```python
from build123d import *

# Parameters (mm, degrees)
F0_R     = 7.5
F0_R_2   = 6.5
F1_DEPTH = 70
F2_R     = 8
F3_DEPTH = 100
F4_R     = 2


with BuildPart() as f1:
    # F0 (on Top) → F1 (new body)
    with BuildSketch(Plane.XY):
        Circle(F0_R)
        Circle(F0_R_2, mode=Mode.SUBTRACT)
    extrude(amount=F1_DEPTH)

    # F2 (on face) → F3 (join)
    with BuildSketch(Plane(origin=(0, 0, 0), x_dir=(1, 0, 0), z_dir=(0, 0, -1))):
        Circle(F2_R)
    extrude(amount=F3_DEPTH)

    # F4
    f4_edges = [f1.edges().sort_by_distance(p)[0] for p in [
        (-8, 0, -100),
    ]]
    fillet(f4_edges, radius=F4_R)


solid = f1.part
```
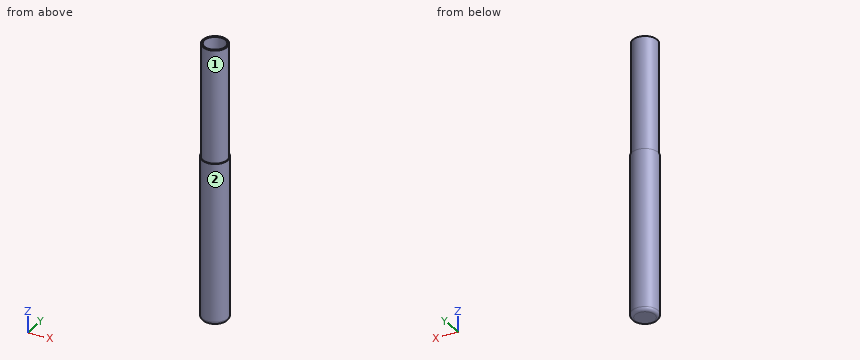
Input: part model. Units: mm. Frame: model coordinates. Face numbers are marked on the shaded views. A direction names the side the tool comes from. Coordinates: 2 decimals unless noted, no trailing zeros. Loops run counter-clockwise (first coordinate to the right, second up) from the corner with the lowest first, then second, coordinate; pieces in that order, holes last.
Q1. Contact query for flat-ended pins moving along their axis: pin 1 (1 mm diameter, centred on y = 4, z = -83, fed in from -X); pin 2 (1.5 mm diameter, centred on x = -3, z = 34, fed in from -Y); pin 3 (2 mm diameter, centred on x = 6, z = -53, fed in from +Y) (3 decimals). Output: stop coordinate, or through.
Results are:
pin 1: stops at x = -7.19
pin 2: stops at y = -7.15
pin 3: stops at y = 6.245
Q2. Line query: line 1 along Y through (x, z) = (0, 14); line 2 along Z through (x, y) = (3.5, -2); line 3 along X through (y, z) = (-2.25, 20). Output: solid intervals per line, ascending.
Results are:
line 1: y = -7.5 to -6.5, 6.5 to 7.5
line 2: z = -100 to 0
line 3: x = -7.15 to -6.1, 6.1 to 7.15
Q3. Section C-C, the plane z = 30. Return the cut outline in (x, y), and give its area (3 significant figures).
Results are:
outline: circle Ø15 at (0, 0); hole circle Ø13 at (0, 0)
area: 44.0 mm2
Q4. Section A-A, the plane x = 0. Return the cut outline in (y, z).
Results are:
outline: (-8, -98) arc R2 ccw to (-6, -100) - (6, -100) arc R2 ccw to (8, -98) - (8, 0) - (7.5, 0) - (7.5, 70) - (6.5, 70) - (6.5, 0) - (-6.5, 0) - (-6.5, 70) - (-7.5, 70) - (-7.5, 0) - (-8, 0) - close
Q5. Section D-D, the plane z = -12. Return the cut outline in (x, y), and give its area (3 significant figures).
Results are:
outline: circle Ø16 at (0, 0)
area: 201 mm2
Q6. Set-up query: the marked faces 1 and 2. Return all of +Z, -Z, +X, -X, +Y, -Y with unobstructed straight access to the full face (end or side cutting, diameter ignored); none if empty.
Results are:
face 1: +Z
face 2: +Z, -Z
